Verification items for the finished model (mm, model axes). A direction names the side the tool comes from. Round coordinates to 2 decimals unless told otherwise and drop trailing zeros. Order: outer loops, then holes, each group sorted by start corner. A loop starts at its lowest first (then second) coordinate and runs counter-clockwise, first axis right, second up. Notation, with made-up numbers: M -8,42.5 L 41,42.5 A31 ccw 41,76.5 Z; hole C -1,-19 d4. An arc over 180 degrees is marked long. Use one line per item in the form item = value. Start each with the question number.
Item 1: Cross-section at C-C on y = -2. Enter the section's corners in (x, z), then the cut area to 3 significant figures.
Item 2: Go/stop test with flat-tipped pins: pin 1 Ø10 at (x, z) = (17, 12.5) entering from +Y; pin 2 Ø2 at (x, y) = (13.5, 19) entering from +Z; pin 3 Ø1.5 at (x, y) = (-28, 17.5) entering from +Z; pin 4 Ø8 at (y, z) = (-7, 14.5) entering from +X. Record where each tip stops, or that it passes through.
Item 3: Thickness scan on probe 1 along Y at (x, z) = (-178, 7.5); probe 2 along Y at (x, z) = (-121, 20.5); probe 3 along Z at (x, y) = (188, 4). Record the ranges inside material, lowest first. Write a range as [from, to].
Item 4: Cross-section at B-B on x = 170.5. Enter the section's corners in (y, z).
Item 5: Cross-section at D-D on y = 25.5. Enter the section's corners in (x, z), then the cut area to 3 significant figures.
Item 6: Cross-section at A-A on z = 11.5. Enter the section's corners in (x, y).
Item 7: Tool access check on faces 1 (the flat face through (3, -13, 15)), 2 (the flat face through (-240, 4, 1)). Record the directions out of +Z, -Z, +X, -X, +Y, -Y that give a thin tool (end or side, any length) a straight path to the whole face; none if there is none.
Autodesk Inventor part; units mm, degrees
ref_plane "YZ Plane" through (0, 0, 0) normal (1, 0, 0) x (0, 1, 0)
ref_plane "XZ Plane" through (0, 0, 0) normal (0, 1, 0) x (-1, 0, 0)
ref_plane "XY Plane" through (0, 0, 0) normal (0, 0, 1) x (1, 0, 0)
sketch "Sketch5" plane through (240, 34.1511, 16.0697) normal (0, 0.6427876, -0.7660444) x (-1, 0, 0)
  line L0 (0, 0) -> (480, 0)
  line L1 (0, 0) -> (480, 0)
  line L2 (470, 0) -> (463.5542, 15)
  line L3 (470, 0) -> (480, -23.2711)
  line L4 (0, -23.2711) -> (480, -23.2711)
  line L5 (0, -23.2711) -> (10, 0)
  line L6 (10, 0) -> (16.4458, 15)
  line L7 (16.4458, 15) -> (463.5542, 15)
  line L8 (240, -23.2711) -> (240, 0) construction
  point P0 (240, -36.4907)
  point P1 (10, 0)
  point P2 (470, 0)
  dimension "d32" = 10
  dimension "d33" = 15
sketch "Sketch1" plane through (0, 0, 0) normal (0, 0, 1) x (1, 0, 0)
  line L0 (-240, -15) -> (240, -15)
  line L1 (240, -15) -> (240, 15)
  line L2 (240, 15) -> (-240, 15)
  line L3 (-240, 15) -> (-240, -15)
  line L4 (-240, -15) -> (240, 15) construction
  line L5 (240, -15) -> (-240, 15) construction
  point P0 (0, 0)
  dimension "d0" = 480
  dimension "d1" = 30
extrude "Plate1" add sketch "Sketch1" along normal blind 2
sketch "Sketch2" plane through (0, 0, 0) normal (0, 0, -1) x (-1, 0, 0)
  line L0 (-220, 5) -> (-20, 5) construction
  line L1 (-20, 5) -> (-20, -15) construction
  line L2 (-20, -15) -> (-220, -15) construction
  line L3 (-220, -15) -> (-220, 5) construction
  line L4 (-240, 15) -> (240, 15)
  line L5 (-240, -15) -> (-240, 15)
  point P0 (0, 0)
  dimension "d6" = 200
  dimension "d9" = 20
  dimension "d10" = 10
  dimension "d11" = 20
mark "Mark1"
sketch "Sketch3" plane through (240, -13, 0) normal (0, -1, 0) x (1, 0, 0)
  line L0 (-480, 0) -> (0, 0)
  line L1 (0, 0) -> (0, 25)
  line L2 (0, 25) -> (-480, 25)
  line L3 (-480, 25) -> (-480, 0)
edge flange "Flange1" height 25 angle 90 thickness 2 bend radius 2.75 thickness toward (0, -1, 0) relief round relief width 2 relief depth 1 edges at (0, -15, 2) wall of the first edge with corners at (-240, -13, 0) (240, -13, 0) (240, -13, 25) (-240, -13, 25)
bend "Bend1"
corner "Corner1"
sketch "Sketch4" plane through (-240, 13.7144, 1.5321) normal (0, 0.6427876, -0.7660444) x (-1, 0, 0)
  line L0 (-480, 0) -> (0, 0)
  line L1 (0, 0) -> (0, 25)
  line L2 (0, 25) -> (-480, 25)
  line L3 (-480, 25) -> (-480, 0)
edge flange "Flange2" height 25 angle 40 thickness 2 bend radius 2.75 thickness toward (0, 0.6427876, -0.7660444) relief round relief width 2 relief depth 1 edges at (0, 15, 2) wall of the first edge with corners at (240, 13.7144, 1.5321) (-240, 13.7144, 1.5321) (-240, 32.8655, 17.6018) (240, 32.8655, 17.6018)
bend "Bend2"
corner "Corner2"
sheet face with bend "Face2" sketch "Sketch5" thickness 2 toward (0, -0.6427876, 0.7660444) bend radius 2.75 contours L6 L7 L2 L0
bend "Bend3"
equation "\"d2\" = Thickness"
equation "\"d12\" = BendReliefWidth"
equation "\"d13\" = BendReliefDepth"
equation "\"d14\" = MinimumRemnant"
equation "\"d15\" = TransitionRadius"
equation "\"d18\" = BendRadius"
equation "\"d19\" = CornerReliefSize"
equation "\"d20\" = GapSize"
equation "\"d21\" = JacobiRadiusSize"
equation "\"d22\" = BendReliefWidth"
equation "\"d23\" = BendReliefDepth"
equation "\"d24\" = MinimumRemnant"
equation "\"d25\" = TransitionRadius"
equation "\"d28\" = BendRadius"
equation "\"d29\" = CornerReliefSize"
equation "\"d30\" = GapSize"
equation "\"d31\" = JacobiRadiusSize"
equation "\"d34\" = BendRadius"
equation "\"d37\" = MinimumRemnant"
equation "\"d35\" = BendReliefWidth"
equation "\"d36\" = BendReliefDepth"
equation "\"d38\" = TransitionRadius"
equation "\"BendReliefWidth\" = Thickness"
equation "\"BendReliefDepth\" = 0.5 * Thickness"
equation "\"CornerReliefSize\" = 4 * Thickness"
equation "\"MinimumRemnant\" = 2 * Thickness"
equation "\"TransitionRadius\" = BendRadius"
equation "\"JacobiRadiusSize\" = BendRadius"
equation "\"GapSize\" = Thickness"
properties part number "TRM 024 top damper" material "AISI 304"
Output values:
q1.outline = M -240,0 L 240,0 L 240,2 L -240,2 Z
q1.area = 960 mm2
q2.pin_1 = 35.86
q2.pin_2 = 6.81
q2.pin_3 = 5.34
q2.pin_4 = through
q3.probe_1 = [-15, -13], [20.83, 23.94]
q3.probe_2 = [-15, -13], [36.32, 39.43]
q3.probe_3 = [0, 2]
q4.outline = M -15,4.75 A4.75 ccw -10.25,0 L 13.27,0 A4.75 ccw 16.32,1.11 L 34.15,16.07 L 45.64,25.71 L 44.36,27.24 L 32.87,17.6 L 15.04,2.64 A2.75 cw 13.27,2 L -10.25,2 A2.75 cw -13,4.75 L -13,25 L -15,25 Z
q5.outline = M -240,8.81 L 240,8.81 L 240,11.42 L -240,11.42 Z
q5.area = 1,250 mm2
q6.outline = M -240,-15 L 240,-15 L 240,-13 L -240,-13 Z; M -240,25.59 L 240,25.59 L 240,28.71 L -240,28.71 Z
q7.face_1 = +Z, +X, -X
q7.face_2 = +Z, -Z, -X, +Y, -Y
